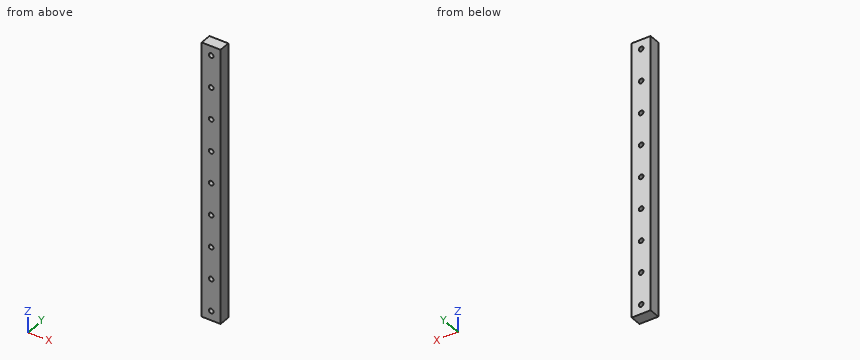
from build123d import *

# Parameters (mm, degrees)
SKETCH1_W           = 10
SKETCH1_H           = 146
BOSS_EXTRUDE1_DEPTH = 6
CUT_EXTRUDE1_REACH  = 75.417
SKETCH2_R           = 1.25
LPATTERN1_COUNT     = 9
LPATTERN1_PITCH     = 17


with BuildPart() as part:
    # Sketch1 → Boss-Extrude1 (new body)
    with BuildSketch(Plane(origin=(0, 0, 0), x_dir=(1, 0, 0), z_dir=(0, 1, 0))):
        Rectangle(SKETCH1_W, SKETCH1_H)
    extrude(amount=BOSS_EXTRUDE1_DEPTH)

    # Sketch2 → Cut-Extrude1 (cut, up to next)
    with BuildSketch(Plane(origin=(0, 6, 0), x_dir=(1, 0, 0), z_dir=(0, 1, 0)), mode=Mode.PRIVATE) as cut_extrude1_sk1:
        with Locations(Location((0, 68, 0), (0, 0, 270))):
            Circle(SKETCH2_R)
    cut_extrude1_tool1 = extrude(cut_extrude1_sk1.sketch, amount=-CUT_EXTRUDE1_REACH, mode=Mode.PRIVATE) & part.part
    cut_extrude1 = cut_extrude1_tool1.solids().sort_by_distance((0, 6, -68))[0]
    add(cut_extrude1, mode=Mode.SUBTRACT)

    # LPattern1: Cut-Extrude1 ×9
    with Locations(*[(0, 0, i * LPATTERN1_PITCH) for i in range(1, LPATTERN1_COUNT)]):
        add(cut_extrude1, mode=Mode.SUBTRACT)


solid = part.part
Work out the finished part from the listing and answer in its coordinate system (mm). Round coordinates to 2 decimals unless told otherwise and drop trailing zeros. Write each loop counter-clockwise with the first axis right and the second up, starting at its lowest first coordinate (ties: lowest second). Pieces come first, ordered by that corner, then holes. Notation, with made-up numbers: (23, 16.5) - (80, 16.5) arc R15 ccw to (80, 28.5) - close; hole circle Ø10 at (-4, 87). An arc over 180 degrees is marked (long way). Answer in a Markdown table with one row per item. Add a question column.
1. A cutting plane is placed at A-A, the plane z = 68. Determine the outline of the cut face in (x, y).
2. Find the intervals of material crossed by line 1 along X through (y, z) = (4.1, -17); line 2 along X through (y, z) = (2.9, -50.5), in increasing order. Write a range as from..to.
3. A cutting plane is placed at B-B, the plane y = 1.95. Count the separate pieces of the cut face and the enclosed holes in it, and give its area (3 significant figures).
Worked out:
| question | item | result |
|---|---|---|
| 1 | outline | (-5, 0) - (-1.25, 0) - (-1.25, 6) - (-5, 6) - close; (1.25, 0) - (5, 0) - (5, 6) - (1.25, 6) - close |
| 2 | line 1 | -5..-1.25, 1.25..5 |
| 2 | line 2 | -5..-1.15, 1.15..5 |
| 3 | separate pieces | 1 |
| 3 | enclosed holes | 9 |
| 3 | area | 1,420 mm^2 |
